Here's the drawing with two shaded views (mm, measured from the low corner). I have some questions. A direction names the side the tool comes from. Give positions to 0.01 mm unless a question says otherwise; leave off trailing zeros. Write each loop counter-clockwise with the first axis right and the second up, starting at its lowest first coordinate (ties: lowest second). Pieces come first, ordered by that corner, then holes. Notation, with made-up numbers: M 61.5,-31.5 L 88.5,-31.5 A23 ccw 88.5,-21.5 Z; hole C 31,-16.75 d4. An arc over 180 degrees is marked long. Use one line per item in the form item = value.
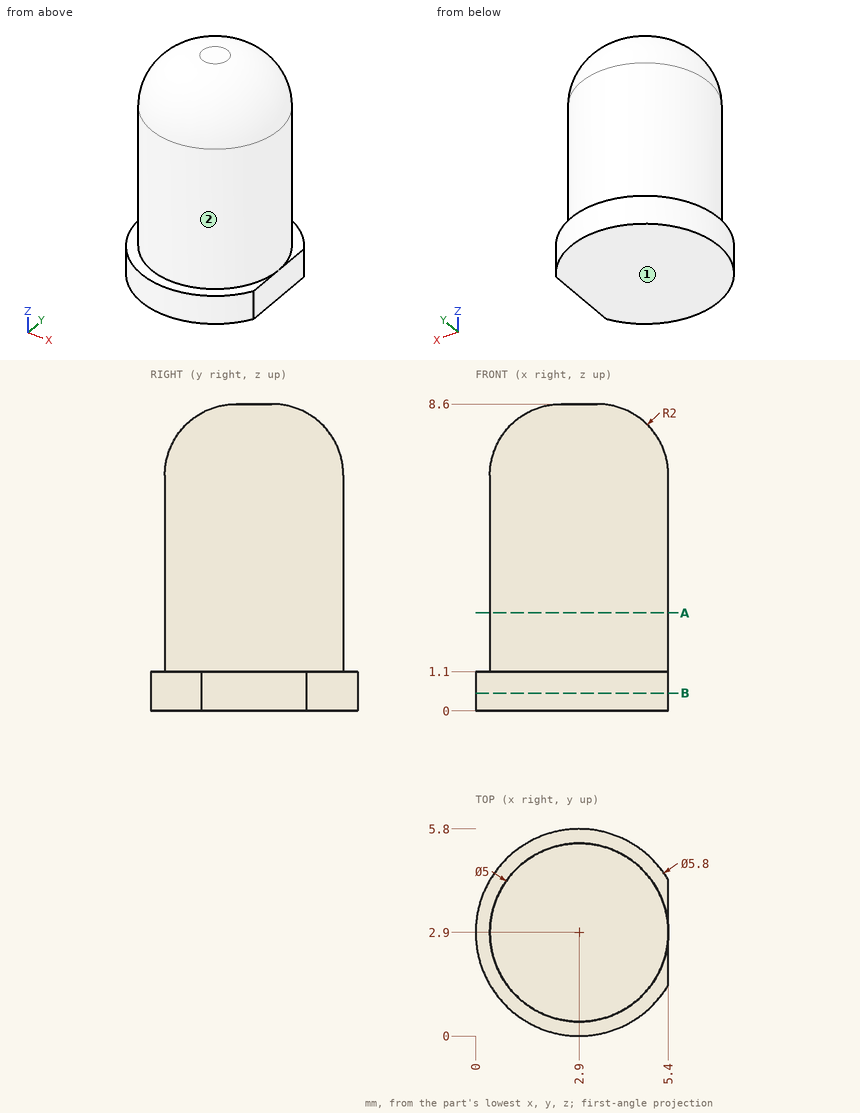
1) For the marked faces 1 and 2, which set-ups out of +Z, -Z, +X, -X, +Y, -Y let a thin tool reach every point of the face, with its end or its side?
Checked values:
face_1 = -Z, +X, -X, +Y, -Y
face_2 = +Z
2) I want a section at B-B, the plane z = 0.5. Please give me the cut outline in (x, y), plus the area to 3 significant figures.
Checked values:
outline = M 5.4,1.43 L 5.4,4.37 A2.9 ccw long Z
area = 25.6 mm2
3) I want a section at A-A, the plane z = 2.75. Please give me the cut outline in (x, y).
Checked values:
outline = C 2.9,2.9 d5
4) If I drill on L1, parallel to Z at x = 2.15, y = 5.45; L2, parallel to Y at x = 2.05, z = 0.5; L3, parallel to Z at x = 4.2, y = 3.1, over which ranges is the centre line in solid material (lowest first)?
Checked values:
L1 = 0 to 1.1
L2 = 0.13 to 5.67
L3 = 0 to 8.43
5) For pin 1 Ø1 at (x, y) = (3.5, 1.5) entering from +Z; pin 2 Ø1.5 at (x, z) = (1, 6.5) entering from -Y, each with a flat end and sliding along its axis, tell me the tip position at first contact or that it passes through.
Checked values:
pin_1 = 8.53
pin_2 = 0.68
